Could you check a few things on this model? Use its own coordinates, in mm. A direction names the side the tool comes from. Round coordinates to 2 decimals unless told otherwise and drop trailing zeros. Loops run counter-clockwise (first coordinate to the right, second up) from the corner with the lowest first, then second, coordinate; pieces in that order, holes last.
from build123d import *

# Parameters (mm, degrees)
F0_R     = 11.90625
F1_DEPTH = 7.14375
F2_R     = 13.97
F3_DEPTH = 7.14375
F5_DEPTH = 25.4


with BuildPart() as f1:
    # F0 (on Top) → F1 (new body)
    with BuildSketch(Plane.XY):
        Circle(F0_R)
    extrude(amount=-F1_DEPTH)

    # F2 (on Top) → F3 (join)
    with BuildSketch(Plane.XY):
        Circle(F2_R)
    extrude(amount=F3_DEPTH)

    # F4 (on face) → F5 (cut)
    with BuildSketch(Plane.XY.offset(7.14375)):
        with BuildLine():
            ThreePointArc((2.38125, 2.100065), (0.198828, 3.168768), (-2.100065, 2.38125))
            ThreePointArc((-2.100065, 2.38125), (-2.245064, 2.245064), (-2.38125, 2.100065))
            Line((-2.38125, 2.100065), (-2.38125, -2.100065))
            ThreePointArc((-2.38125, -2.100065), (0, -3.175), (2.38125, -2.100065))
            Line((2.38125, -2.100065), (2.38125, 2.100065))
        make_face()
    extrude(amount=-F5_DEPTH, mode=Mode.SUBTRACT)


solid = f1.part
Item 1: If we section it at B-B, the plane y = 0: Please give me the cut outline in (x, z), then the cut area to 3 significant figures.
Results list:
outline: (-13.97, 0) - (-11.91, 0) - (-11.91, -7.14) - (-2.38, -7.14) - (-2.38, 7.14) - (-13.97, 7.14) - close; (2.38, -7.14) - (11.91, -7.14) - (11.91, 0) - (13.97, 0) - (13.97, 7.14) - (2.38, 7.14) - close
area: 302 mm2
Item 2: If we section it at A-A, the plane x = 0: Please give me the cut outline in (y, z) (3 decimals), then the cut area to 3 significant figures.
Results list:
outline: (-13.97, 0) - (-11.906, 0) - (-11.906, -7.144) - (-3.175, -7.144) - (-3.175, 7.144) - (-13.97, 7.144) - close; (3.175, -7.144) - (11.906, -7.144) - (11.906, 0) - (13.97, 0) - (13.97, 7.144) - (3.175, 7.144) - close
area: 279 mm2
Item 3: We'd pull the mould along Y, two halves only. Please class faces 4 (the flat face through (10.3, 6.3, 0)), 5 (the cylindrical face through (-1.82, 13.85, 3.52)), 6 (the cylindrical face through (-0.038, -3.175, 0.1)): released by +Y, released by -Y, zero draft, split by the parting line, or undercut.
Results list:
face 4: zero draft
face 5: split by the parting line
face 6: undercut
Item 4: For faces 1 (the flat face through (2.381, 0, 0)), 2 (the cylindrical face through (-9.45, -7.24, -3.52)), 3 (the flat face through (-3, 0, -7.144)), which set-ups out of +Z, -Z, +X, -X, +Y, -Y let a thin tool reach every point of the face, with its end or its side?
Results list:
face 1: +Z, -Z
face 2: -Z
face 3: -Z, +X, -X, +Y, -Y
Item 5: If I drill on line 1 along X through (y, z) = (-0.25, -2.25); line 2 along Z through (x, y) = (5.75, 12.25); line 3 along Y through (x, z) = (-9.75, -3.25), over which ranges is the centre line in solid material (lowest first)?
Results list:
line 1: x = -11.9 to -2.38, 2.38 to 11.9
line 2: z = 0 to 7.14
line 3: y = -6.83 to 6.83
Item 6: If we section it at D-D, the plane y = 10: Please give me the cut outline in (x, z).
Results list:
outline: (-9.76, 0) - (-6.46, 0) - (-6.46, -7.14) - (6.46, -7.14) - (6.46, 0) - (9.76, 0) - (9.76, 7.14) - (-9.76, 7.14) - close
Item 7: Will these pins go through, and if not, where does the flat tip stop? pin 1 (5 mm diameter, centred on y = -8.5, z = 0.5, fed in from -X); pin 2 (3 mm diameter, centred on y = -9, z = 2.5, fed in from -X); pin 3 (4.5 mm diameter, centred on y = -1, z = -3, fed in from -X); pin 4 (4.5 mm diameter, centred on y = 0, z = -2, fed in from +X).
Results list:
pin 1: stops at x = -12.62
pin 2: stops at x = -11.79
pin 3: stops at x = -11.91
pin 4: stops at x = 13.97
